Read the model definition and answer for the solid it produces. Units are mm, in the model's axes. Face numbers are marked on the shaded views. Give positions to 0.01 mm unless a question says otherwise; leave off trailing zeros. Order: outer loops, then holes, each group sorted by start corner. A loop starts at its lowest first (then second) coordinate and runs counter-clockwise, first axis right, second up. Notation, with made-up numbers: (46, 4) - (98, 4) arc R18 cw to (98, 33) - close; hole circle Ø5 at (64, 29). An arc over 180 degrees is marked (long way). Use a Markdown table: item, result. Add a question column.
1. For a pull along Y with two mould halves and no side action, classify the marked faces 1, 2, 3 and 4 as released by +Y, released by -Y, zero draft, split by the parting line, or undercut.
2. A cutting plane is placed at A-A on x = 0. Determine the outline of the cut face in (y, z), and give its area (3 significant figures).
3. A cutting plane is placed at C-C on x = -29. Determine the outline of the cut face in (y, z).
4. Flat-ended cylindrical pins translate along their axes: P1, Ø1.9, axis at y = -149, z = 75, coming from the -X side; P2, Ø10, axis at y = -18.5, z = 24, coming from the -X side; P3, Ø3, axis at x = -28.5, y = -105, coming from the +Z side. Find the tip coordinate at first contact, or state that the pin passes through.
5. Consider L1, parallel to Y at x = 0, z = 73.25; L2, parallel to Z at x = -20.5, y = -53; L3, parallel to Y at x = 8.5, z = 73.5. Determine where each line is inside the solid, lowest interval first.
6. A cutting plane is placed at B-B on y = -9. Determine the outline of the cut face in (x, z), and give its area (3 significant figures).
7. A cutting plane is placed at D-D on y = -120.5. Determine the outline of the cut face in (x, z), and give its area (3 significant figures).
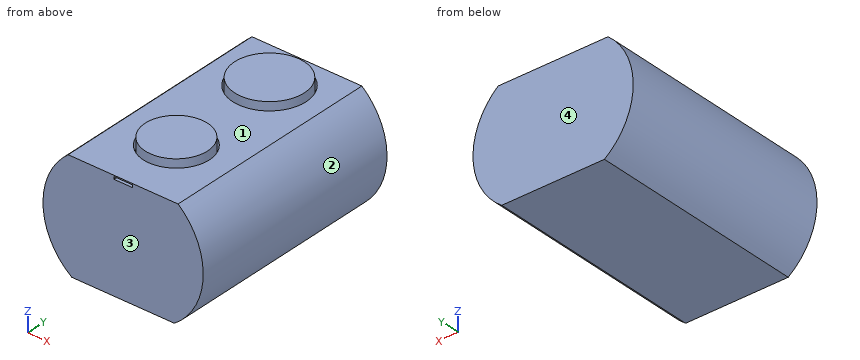
```python
from build123d import *

# Parameters (mm, degrees)
F1_DEPTH  = 152.4
F2_R      = 35.861849
F2_R_2    = 34.861464
F3_DEPTH  = 7.62
F4_R      = 25.4
F5_DEPTH  = 7.62
F6_R      = 24.13
F7_DEPTH  = 12.7
F8_R      = 22.86
F9_DEPTH  = 7.62
F10_R     = 21.59
F11_DEPTH = 12.7
F12_W     = 12.7
F12_H     = 1.719565
F13_DEPTH = 12.7


with BuildPart() as f1:
    # F0 (on Front) → F1 (new body)
    with BuildSketch(Plane.XZ):
        with BuildLine():
            Line((-35.56, 0), (0, 0))
            Line((0, 0), (0, 76.2))
            Line((0, 76.2), (-38.1, 76.2))
            ThreePointArc((-38.1, 76.2), (-55.485641, 37.478145), (-35.56, 0))
        make_face()
        with BuildLine():
            Line((0, 76.2), (0, 0))
            Line((0, 0), (35.56, 0))
            ThreePointArc((35.56, 0), (55.485641, 37.478145), (38.1, 76.2))
            Line((38.1, 76.2), (0, 76.2))
        make_face()
    extrude(amount=F1_DEPTH)

    # F2 (on face) → F3 (cut)
    with BuildSketch(Plane.XY.offset(76.2)):
        with Locations((0, -520.644426)):
            Circle(F2_R)
        with Locations((0, -297.697842)):
            Circle(F2_R_2)
    extrude(amount=-F3_DEPTH, mode=Mode.SUBTRACT)

    # F4 (on face) → F5 (cut)
    with BuildSketch(Plane.XY.offset(76.2)):
        with Locations((0, -31.021852)):
            Circle(F4_R)
    extrude(amount=-F5_DEPTH, mode=Mode.SUBTRACT)

    # F6 (on face) → F7 (join)
    with BuildSketch(Plane.XY.offset(68.58)):
        with Locations((0, -31.021852)):
            Circle(F6_R)
    extrude(amount=F7_DEPTH)

    # F8 (on face) → F9 (cut)
    with BuildSketch(Plane.XY.offset(76.2)):
        with Locations((0, -108.224646)):
            Circle(F8_R)
    extrude(amount=-F9_DEPTH, mode=Mode.SUBTRACT)

    # F10 (on face) → F11 (join)
    with BuildSketch(Plane.XY.offset(68.58)):
        with Locations((0, -108.224646)):
            Circle(F10_R)
    extrude(amount=F11_DEPTH)

    # F12 (on face) → F13 (cut)
    with BuildSketch(Plane.XZ.offset(152.4)):
        with Locations((0, 74.519782)):
            Rectangle(F12_W, F12_H)
    extrude(amount=-F13_DEPTH, mode=Mode.SUBTRACT)


solid = f1.part
```
Output values:
| question | item | result |
|---|---|---|
| 1 | face 1 | undercut |
| 1 | face 2 | zero draft |
| 1 | face 3 | released by -Y |
| 1 | face 4 | released by +Y |
| 2 | outline | (-152.4, 0) - (0, 0) - (0, 76.2) - (-5.62, 76.2) - (-5.62, 68.58) - (-6.89, 68.58) - (-6.89, 81.28) - (-55.15, 81.28) - (-55.15, 68.58) - (-56.42, 68.58) - (-56.42, 76.2) - (-85.36, 76.2) - (-85.36, 68.58) - (-86.63, 68.58) - (-86.63, 81.28) - (-129.81, 81.28) - (-129.81, 68.58) - (-131.08, 68.58) - (-131.08, 76.2) - (-152.4, 76.2) - (-152.4, 75.38) - (-139.7, 75.38) - (-139.7, 73.66) - (-152.4, 73.66) - close |
| 2 | area | 12,000 mm² |
| 3 | outline | (-152.4, 0) - (0, 0) - (0, 76.2) - (-152.4, 76.2) - close |
| 4 | P1 | x = -40.52 |
| 4 | P2 | x = -54.45 |
| 4 | P3 | z = 76.2 |
| 5 | L1 | -152.4 to -131.08, -129.81 to -86.63, -85.36 to -56.42, -55.15 to -6.89, -5.62 to 0 |
| 5 | L2 | 0 to 76.2 |
| 5 | L3 | -152.4 to -129.45, -128.07 to -88.38, -87 to -54.96, -53.61 to -8.44, -7.09 to 0 |
| 6 | outline | (-38.1, 76.2) arc R48.26 ccw to (-35.56, 0) - (35.56, 0) arc R48.26 ccw to (38.1, 76.2) - (12.66, 76.2) - (12.66, 68.58) - (9.86, 68.58) - (9.86, 81.28) - (-9.86, 81.28) - (-9.86, 68.58) - (-12.66, 68.58) - (-12.66, 76.2) - close |
| 6 | area | 7,660 mm² |
| 7 | outline | (-38.1, 76.2) arc R48.26 ccw to (-35.56, 0) - (35.56, 0) arc R48.26 ccw to (38.1, 76.2) - (19.28, 76.2) - (19.28, 68.58) - (17.76, 68.58) - (17.76, 81.28) - (-17.76, 81.28) - (-17.76, 68.58) - (-19.28, 68.58) - (-19.28, 76.2) - close |
| 7 | area | 7,760 mm² |
